The listing builds one solid part. Answer for the finished solid, in the listing's coordinates (mm). Give positions to 0.01 mm unless a question says otherwise; leave off trailing zeros. Order: outer loops, then holes, each group sorted by start corner. A loop starts at its lowest first (then second) coordinate and runs counter-clockwise, first axis right, second up. Notation, with made-up numbers: (26, 61) - (56, 61) arc R33 ccw to (56, 100) - close; hole circle Ø11 at (-34.75, 75). An arc over 180 degrees is marked (long way). Write each question's results on one line, items separated by ' | '. Start each with the question number.
1. Find the intervals of material crossed by L1, parallel to Y at x = -19, z = 2; L2, parallel to Z at x = -14, y = 37; L3, parallel to Z at x = -17, y = -3.5, in increasing order.
2. Flat-ended cylindrical pins translate along their axes: pin 1 (8 mm diameter, centred on x = 13, z = 9.5, fed in from +Y); pin 2 (3 mm diameter, centred on x = -13, y = 10.5, fed in from +Z); pin 3 (4 mm diameter, centred on x = -1, z = 7, fed in from -Y). Find the tip coordinate at first contact, or state that the pin passes through.
3. Section A-A (z = 2) is taken. Give the vertices of the cut face in (x, y).
from build123d import *

# Parameters (mm, degrees)
F0_W     = 43
F0_H     = 76
F1_DEPTH = 12
F5_DEPTH = 25


with BuildPart() as f1:
    # F0 (on Top) → F1 (new body)
    with BuildSketch(Plane.XY):
        Rectangle(F0_W, F0_H)
    extrude(amount=F1_DEPTH)

    # F3 (on Right) → F4 (revolve)
    with BuildSketch(Plane.YZ):
        with BuildLine():
            Line((-44.1283285618, 12), (9.5, 12))
            Line((9.5, 12), (9.5, 13))
            add(Edge.make_bspline(
                [(9.5, 13), (7.2259709093, 12.9839292355), (3.8143336998, 17.3923027091), (0.0559037939, 10.903183264), (-3.8044043801, 16.6240806281), (-8.5884909723, 11.3816701472), (-12.7677373796, 15.9904534972), (-20.2609269277, 11.5681742154), (-27.8215516911, 15.5335878921), (-38.0023366763, 12.8770661415), (-44.1283285618, 12)],
                knots=[0, 0, 0, 0, 0.1201180453, 0.2223436831, 0.3231585069, 0.43149146, 0.5353595882, 0.666400511, 0.8015197875, 1, 1, 1, 1], degree=3))
        make_face()
    revolve(axis=Axis((0, 9.5, 12.5), (0, 0, 1)))

    # F5 (cut): a face of the model
    f5_faces = [f1.faces().sort_by_distance(p)[0] for p in [
        (0, 61.6114903702, 12),
    ]]
    extrude(f5_faces, amount=-F5_DEPTH, mode=Mode.SUBTRACT)


solid = f1.part
Reported:
1) L1: -38 to 38 | L2: 0 to 12.94 | L3: 0 to 14.22
2) pin 1: y = 38 | pin 2: z = 14.79 | pin 3: y = -38
3) outline: (-21.5, -38) - (21.5, -38) - (21.5, 38) - (-21.5, 38) - close
